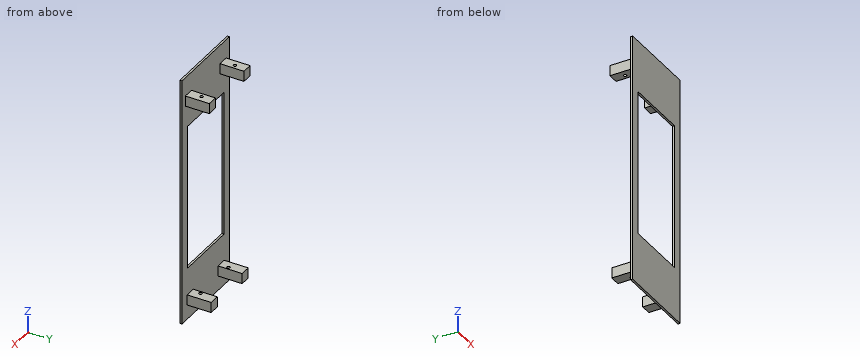
from build123d import *

# Parameters (mm, degrees)
SKETCH_W        = 39
SKETCH_H        = 1
PAD_DEPTH       = 120
SKETCH001_W     = 5
SKETCH001_H     = 5
PAD001_DEPTH    = 11.5
SKETCH003_R     = 0.75
POCKET_DEPTH    = 5
SKETCH002_R     = 0.75
POCKET001_DEPTH = 5
SKETCH004_W     = 30
SKETCH004_H     = 70
POCKET002_DEPTH = 5


with BuildPart() as part:
    # Sketch → Pad (new body)
    with BuildSketch(Plane.XY):
        with Locations((19.5, 0.5)):
            Rectangle(SKETCH_W, SKETCH_H)
    extrude(amount=PAD_DEPTH)

    # Sketch001 → Pad001 (new body)
    with BuildSketch(Plane(origin=(0, 1, 0), x_dir=(-1, 0, 0), z_dir=(0, 1, 0))):
        with Locations((-33.75, 108.5)):
            Rectangle(SKETCH001_W, SKETCH001_H)
        with Locations((-5.25, 108.5)):
            Rectangle(SKETCH001_W, SKETCH001_H)
        with Locations((-32.25, 9.5)):
            Rectangle(SKETCH001_W, SKETCH001_H)
        with Locations((-6.75, 9.5)):
            Rectangle(SKETCH001_W, SKETCH001_H)
    extrude(amount=PAD001_DEPTH)

    # Sketch003 → Pocket (cut)
    with BuildSketch(Plane.XY.offset(111)):
        with Locations((5.75, 7)):
            Circle(SKETCH003_R)
        with Locations((33.25, 7)):
            Circle(SKETCH003_R)
    extrude(amount=-POCKET_DEPTH, mode=Mode.SUBTRACT)

    # Sketch002 → Pocket001 (cut)
    with BuildSketch(Plane(origin=(0, 0, 7), x_dir=(1, 0, 0), z_dir=(0, 0, -1))):
        with Locations((31, -5.2)):
            Circle(SKETCH002_R)
        with Locations((8, -5.2)):
            Circle(SKETCH002_R)
    extrude(amount=-POCKET001_DEPTH, mode=Mode.SUBTRACT)

    # Sketch004 → Pocket002 (cut)
    with BuildSketch(Plane(origin=(0, 1, 0), x_dir=(-1, 0, 0), z_dir=(0, 1, 0))):
        with Locations((-19.5, 60)):
            Rectangle(SKETCH004_W, SKETCH004_H)
    extrude(amount=-POCKET002_DEPTH, mode=Mode.SUBTRACT)


solid = part.part
Verification items for the finished model (mm, model axes). Give positions to 0.01 mm unless a question says otherwise; leave off trailing zeros. Write each loop counter-clockwise with the first axis right and the second up, starting at its lowest first coordinate (ties: lowest second). Pieces come first, ordered by that corner, then holes. Notation, with made-up numbers: M -30,48.25 L -9,48.25 A22 ccw -9,55.25 Z; hole C 38.25,34.25 d2. An arc over 180 degrees is marked long. Use CSV: the item, a comma, the result in double quotes.
1) Cross-section at A-A (y = 3.25). Enter the section's corners in (x, z).
Final values:
outline,"M 2.75,106 L 7.75,106 L 7.75,111 L 2.75,111 Z; M 4.25,7 L 9.25,7 L 9.25,12 L 4.25,12 Z; M 29.75,7 L 34.75,7 L 34.75,12 L 29.75,12 Z; M 31.25,106 L 36.25,106 L 36.25,111 L 31.25,111 Z"
2) Cross-section at B-B (z = 55.5). Enter the section's corners in (x, y), plus the area to 3 significant figures.
Final values:
outline,"M 0,0 L 4.5,0 L 4.5,1 L 0,1 Z; M 34.5,0 L 39,0 L 39,1 L 34.5,1 Z"
area,"9.00 mm²"
3) Go/stop test with flat-tipped pins: pin 1 Ø12 at (x, z) = (26, 20) entering from +Y; pin 2 Ø2.5 at (y, z) = (4, 9) entering from -X; pin 3 Ø4 at (x, y) = (32.5, 9.5) entering from +Z. Record where each tip stops, or that it passes through.
Final values:
pin 1,"y = 1"
pin 2,"x = 4.25"
pin 3,"z = 111"
4) Cross-section at C-C (x = 15). Enter the section's corners in (y, z), plus the area to 3 significant figures.
Final values:
outline,"M 0,0 L 1,0 L 1,25 L 0,25 Z; M 0,95 L 1,95 L 1,120 L 0,120 Z"
area,"50.0 mm²"
5) Material ranges on line 1 along X through (y, z) = (5.2, 8.6); line 2 along X through (y, z) = (0.75, 79.5); line 3 along Y through (x, z) = (5.75, 109.95), recorded low to high.
Final values:
line 1,"4.25 to 7.25, 8.75 to 9.25, 29.75 to 30.25, 31.75 to 34.75"
line 2,"0 to 4.5, 34.5 to 39"
line 3,"0 to 6.25, 7.75 to 12.5"
6) Cross-section at D-D (z = 99). Enter the section's corners in (x, y), plus the area to 3 significant figures.
Final values:
outline,"M 0,0 L 39,0 L 39,1 L 0,1 Z"
area,"39.0 mm²"
